Input: part model. Units: mm. Frame: model coordinates. A direction names the side the tool comes from. Coordinates: 2 decimals unless noted, no trailing zeros. Order: outer loops, then holes, each group sorted by start corner. A loop starts at its lowest first (then second) coordinate and runs counter-clockwise, first axis right, second up. Notation, with made-up numbers: M -3,60 L 38,60 A16 cw 38,91 Z; hole C 34,33.5 d8. An arc over 180 degrees is marked long. One line per item, written item: value.
```python
from build123d import *

# Parameters (mm, degrees)
SKETCH1_W               = 12
SKETCH1_H               = 7
BOSS_EXTRUDE1_DEPTH     = 3
CUT_EXTRUDE1_DEPTH      = 7
CUT_EXTRUDE2_DEPTH      = 15.212670404
CUT_EXTRUDE2_DEPTH_BACK = 15.212670404
SKETCH4_R               = 1.8
CUT_EXTRUDE3_DEPTH      = 0.8
SKETCH5_W               = 0.519230769
SKETCH5_H               = 2.7
CUT_EXTRUDE4_DEPTH      = 0.4


with BuildPart() as part:
    # Sketch1 → Boss-Extrude1 (new body)
    with BuildSketch(Plane(origin=(0, 0, 0), x_dir=(1, 0, 0), z_dir=(0, 1, 0))):
        with Locations((6, 3.5)):
            Rectangle(SKETCH1_W, SKETCH1_H)
    extrude(amount=BOSS_EXTRUDE1_DEPTH)

    # Sketch2 → Cut-Extrude1 (cut)
    with BuildSketch(Plane.XY):
        Polygon((0, 0), (0.7, 3), (0, 3), align=None)
        Polygon((12, 0), (11.3, 3), (12, 3), align=None)
    extrude(amount=-CUT_EXTRUDE1_DEPTH, mode=Mode.SUBTRACT)

    # Sketch3 → Cut-Extrude2 (cut, two sides: drawn at the far end of the back side and taken through both)
    with BuildSketch(Plane(origin=(0, 0, 0), x_dir=(0, 0, -1), z_dir=(1, 0, 0)).offset(-CUT_EXTRUDE2_DEPTH_BACK)):
        Polygon((0, 0), (0.7, 3), (0, 3), align=None)
        Polygon((7, 3), (6.3, 3), (7, 0), align=None)
    extrude(amount=CUT_EXTRUDE2_DEPTH + CUT_EXTRUDE2_DEPTH_BACK, mode=Mode.SUBTRACT)

    # Sketch4 → Cut-Extrude3 (cut)
    with BuildSketch(Plane.XZ):
        with Locations(Location((6, -3.5, 0), (0, 0, 270))):
            Circle(SKETCH4_R)
    extrude(amount=-CUT_EXTRUDE3_DEPTH, mode=Mode.SUBTRACT)

    # Sketch5 → Cut-Extrude4 (cut)
    with BuildSketch(Plane(origin=(0, 3, 0), x_dir=(1, 0, 0), z_dir=(0, 1, 0))):
        Polygon((3.035523477, 2.141483951), (2.389189343, 4.841483951), (2.921400881, 4.841483951), (3.341112419, 2.986856547), (3.7851629, 4.841483951), (4.493696554, 4.841483951), (4.933420112, 2.955486355), (5.352049919, 4.841483951), (5.885343189, 4.841483951), (5.250908093, 2.141483951), (4.60781915, 2.141483951), (4.137266266, 4.159993566), (3.654273477, 2.141483951), align=None)
        with Locations((6.421881651, 3.491483951)):
            Rectangle(SKETCH5_W, SKETCH5_H)
        Polygon((7.235343189, 2.141483951), (7.235343189, 4.841483951), (7.777831169, 4.841483951), (8.862266266, 3.066363758), (8.862266266, 4.841483951), (9.381497035, 4.841483951), (9.381497035, 2.141483951), (8.822242227, 2.141483951), (7.754573958, 3.888479143), (7.754573958, 2.141483951), align=None)
    extrude(amount=-CUT_EXTRUDE4_DEPTH, mode=Mode.SUBTRACT)


solid = part.part
```
(1) Cut plane C-C on y = 1.95. Output: boundary loops of the cut face in (x, z) (3 decimals).
Data:
outline: M 0.455,-6.545 L 11.545,-6.545 L 11.545,-0.455 L 0.455,-0.455 Z
(2) Ray query, line 1 (Y direction, x = 3.75, z = -4.5); line 2 (Z direction, x = 9.25, y = 2.8); line 3 (Y direction, x = 7, z = -4.5). Return the intervals inside material, ascending. Write a range as from..to.
Data:
line 1: y = 0..2.6
line 2: z = -6.35..-4.84, -2.14..-0.65
line 3: y = 0.8..3
(3) Cut plane A-A on x = 9. Output: boundary loops of the cut face in (y, z).
Data:
outline: M 0,-7 L 3,-6.3 L 3,-4.84 L 2.6,-4.84 L 2.6,-2.14 L 3,-2.14 L 3,-0.7 L 0,0 Z
(4) Draft query along Z for faces 1 (the flat face through (5.916, 1.521, -6.645)), 2 (the flat face through (8, 2.6, -4)), 3 (the flat face through (11.655, 1.479, -3.451)). Return one class per face: released by +Z, released by -Z, zero draft, split by the parting line, or undercut.
Data:
face 1: released by -Z
face 2: undercut
face 3: zero draft
(5) First-contact query: pin 1 (1.5 mm diameter, centred on x = 6, y = 2, fed in from +Z); pin 2 (1 mm diameter, centred on x = 5.5, y = 2.5, fed in from +Z); pin 3 (0.6 mm diameter, centred on x = 6.5, z = -3.5, fed in from +Y). Flat tips, straight axial feed; report the tip coordinate or a pass-through.
Data:
pin 1: stops at z = -0.29
pin 2: stops at z = -0.47
pin 3: stops at y = 3
(6) Access query for faces 4 (the flat face through (0.345, 1.479, -3.451)), 5 (the flat face through (3.8, 2.6, -3.5)), 6 (the cylindrical face through (4.403, 0.394, -4.331)). Directions: +Z, -Z, +X, -X, +Y, -Y. A direction counts if a zero-diameter tool reaches every point of the face in a straight line with its end or side. Return the directions, or none.
Data:
face 4: +Z, -Z, -X, +Y
face 5: +Y
face 6: -Y
(7) Cut plane B-B on z = -5. Output: boundary loops of the cut face in (x, y), plus the area to 3 significant figures.
Data:
outline: M 0,0 L 5.01,0 L 5.01,0.8 L 6.99,0.8 L 6.99,0 L 12,0 L 11.3,3 L 0.7,3 Z
area: 32.3 mm2
(8) Cut plane D-D on z = -2.75. Output: boundary loops of the cut face in (x, y).
Data:
outline: M 0,0 L 4.36,0 L 4.36,0.8 L 7.64,0.8 L 7.64,0 L 12,0 L 11.3,3 L 9.38,3 L 9.38,2.6 L 8.45,2.6 L 8.45,3 L 7.75,3 L 7.75,2.6 L 7.24,2.6 L 7.24,3 L 6.68,3 L 6.68,2.6 L 6.16,2.6 L 6.16,3 L 5.39,3 L 5.39,2.6 L 4.47,2.6 L 4.47,3 L 3.8,3 L 3.8,2.6 L 2.89,2.6 L 2.89,3 L 0.7,3 Z
